Design review of the part built by this model. Coordinates are the model's own, in mm. Face numbers are marked on the shaded views. A direction names the side the tool comes from. Coordinates: 2 decimals unless noted, no trailing zeros. Loops run counter-clockwise (first coordinate to the right, second up) from the corner with the lowest first, then second, coordinate; pieces in that order, holes last. Notation, with made-up numbers: (62, -36) -> (120, -36) arc R3 ccw to (120, -32) -> close; hole circle Ø11 at (-17.5, 60). An arc over 180 degrees is marked (long way). Answer as a JSON object with one key per item and string values.
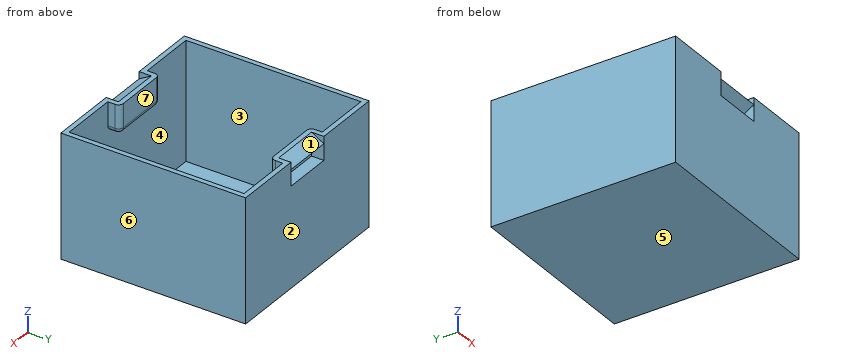
```python
from build123d import *

# Parameters (mm, degrees)
SKETCH_W     = 75
SKETCH_H     = 75
PAD_DEPTH    = 50
SKETCH001_W  = 20
SKETCH001_H  = 10
POCKET_DEPTH = 5
THICKNESS_T  = -2
PAD001_DEPTH = 20


with BuildPart() as part:
    # Sketch → Pad (new body)
    with BuildSketch(Plane.XY):
        Rectangle(SKETCH_W, SKETCH_H)
    extrude(amount=PAD_DEPTH)

    # Sketch001 (on Face2 of Pad) → Pocket (cut)
    with BuildSketch(Plane.XZ.offset(37.5)):
        with Locations((0, 45.5)):
            Rectangle(SKETCH001_W, SKETCH001_H)
    pocket = extrude(amount=-POCKET_DEPTH, mode=Mode.SUBTRACT)

    # Mirrored: Pocket across XZ
    add(pocket.mirror(Plane.XZ), mode=Mode.SUBTRACT)

    # Thickness
    thickness_openings = [part.faces().sort_by_distance(p)[0] for p in [
        (0, 0, 50),
    ]]
    offset(amount=THICKNESS_T, openings=thickness_openings)

    # Sketch002 (on Face11 of Thickness) → Pad001 (join)
    with BuildSketch(Plane.YZ.offset(-10)):
        Polygon((-32.5, 50), (-37.5, 47.113249), (-32.5, 44.226497), align=None)
    pad001 = extrude(amount=PAD001_DEPTH)

    # Mirrored001: Pad001 across XZ
    add(pad001.mirror(Plane.XZ))


solid = part.part
```
1) Add section A-A, the plane z = 9. Give the boundary of the cut face in (x, y).
Completed:
{"outline": "(-37.5, -37.5) -> (37.5, -37.5) -> (37.5, 37.5) -> (-37.5, 37.5) -> close; hole (-35.5, -35.5) -> (35.5, -35.5) -> (35.5, 35.5) -> (-35.5, 35.5) -> close"}
2) The part is to be moulded in two halves that separate along X. For the marked faces 4, 5, 6 and 7, say which applies: pulls with the +X half, pulls with the -X half, needs draft (parallel to the pull), parting line crosses it, or undercut.
Completed:
{"face 4": "undercut", "face 5": "needs draft", "face 6": "pulls with the +X half", "face 7": "undercut"}
3) For the marked faces 1, 2 and 3, list the 3-axis set-ups (+Z, -Z, +X, -X, +Y, -Y) from which the entire face can be reached by the end or side of a thin tool; tool diameter is ignored.
Completed:
{"face 1": "+Z, +Y", "face 2": "+Z, -Z, +X, -X, +Y", "face 3": "+Z"}
4) Wall thickness on probe 1 along Y at (x, z) = (21, 35); probe 2 along Z at (x, y) = (-21, 20): over which ranges is each line inside the solid? List them lowest first.
Completed:
{"probe 1": "-37.5 to -35.5, 35.5 to 37.5", "probe 2": "0 to 2"}
5) Clearance check with flat-ended pins moving along their axes: pin 1 Ø1.5 at (x, y) = (1.5, -34.5) entering from -Z; pin 2 Ø3 at (x, z) = (-3.5, 45) entering from -Y; pin 3 Ø3 at (x, y) = (15, 26.5) entering from +Z; pin 4 Ø5 at (x, z) = (0, 46) entering from +Y. State where each tip first meets the part, or that it passes through.
Completed:
{"pin 1": "z = 0", "pin 2": "y = -36.44", "pin 3": "z = 2", "pin 4": "y = 37.5"}
6) Add section D-D, the plane z = 42. Give the boundary of the cut face in (x, y), and give its area (3 significant figures).
Completed:
{"outline": "(-37.5, -37.5) -> (-10, -37.5) -> (-10, -32.5) -> (10, -32.5) -> (10, -37.5) -> (37.5, -37.5) -> (37.5, 37.5) -> (10, 37.5) -> (10, 32.5) -> (-10, 32.5) -> (-10, 37.5) -> (-37.5, 37.5) -> close; hole (-35.5, -35.5) -> (-12, -35.5) -> (-12, -32.5) arc R2 cw to (-10, -30.5) -> (10, -30.5) arc R2 cw to (12, -32.5) -> (12, -35.5) -> (35.5, -35.5) -> (35.5, 35.5) -> (12, 35.5) -> (12, 32.5) arc R2 cw to (10, 30.5) -> (-10, 30.5) arc R2 cw to (-12, 32.5) -> (-12, 35.5) -> (-35.5, 35.5) -> close", "area": "621 mm²"}
7) Add section B-B, the plane y = 13. Give the boundary of the cut face in (x, z), and give its area (3 significant figures).
Completed:
{"outline": "(-37.5, 0) -> (37.5, 0) -> (37.5, 50) -> (35.5, 50) -> (35.5, 2) -> (-35.5, 2) -> (-35.5, 50) -> (-37.5, 50) -> close", "area": "342 mm²"}
